CAD build for the part. Positions are in the model's coordinates, mm. A direction names the side the tool comes from. Round coordinates to 2 decimals unless told otherwise and drop trailing zeros. Order: outer loops, then holes, each group sorted by start corner. A loop starts at its lowest first (then second) coordinate and runs counter-clockwise, first axis right, second up. Notation, with made-up numbers: (71, -7) - (92, -7) arc R18 ccw to (92, 15) - close; hole circle Ø6 at (56, 12.25). An arc over 180 degrees is marked (long way). Use one line per item in the form item = value. Start each with the question number.
Autodesk Inventor part; units mm, degrees
ref_plane "YZ Plane" through (0, 0, 0) normal (1, 0, 0) x (0, 1, 0)
ref_plane "XZ Plane" through (0, 0, 0) normal (0, 1, 0) x (-1, 0, 0)
ref_plane "XY Plane" through (0, 0, 0) normal (0, 0, 1) x (1, 0, 0)
sketch "Sketch1" plane through (0, 0, 0) normal (0, 0, 1) x (1, 0, 0)
  line L0 (-3.0704, 18.7151) -> (-3.0704, 6.0151)
  line L1 (-3.0704, 6.0151) -> (-6.8804, 6.0151)
  line L2 (-6.8804, 6.0151) -> (-6.8804, -10.4949)
  line L3 (-6.8804, -10.4949) -> (-3.0704, -10.4949)
  line L4 (-3.0704, -10.4949) -> (-3.0704, -16.8449)
  line L5 (-3.0704, -16.8449) -> (-1.8004, -16.8449)
  line L6 (-1.8004, 18.7151) -> (-3.0704, 18.7151)
  line L7 (-1.8004, 18.7151) -> (-1.8004, -16.8449)
  dimension "d0" = 16.51
  dimension "d1" = 12.7
  dimension "d3" = 1.27
  dimension "d8" = 5.08
  dimension "d9" = 6.35
revolve "Revolution1" add sketch "Sketch1" angle 360 about axis through (-1.8004, 18.7151, 0) along (0, -1, 0)
properties part number "roll1"
(1) Which spindle directions (+Z, -Z, +X, -X, +Y, -Y) get a long thin tool onto all of the face, cutting with end or side? Do faces 1 (the cylindrical face through (-1.64, 12.28, -1.26)), 2 (the cylindrical face through (1.944, -2.355, -3.433)), 3 (the cylindrical face through (-1.64, -13.71, -1.26)). Say none if no direction does.
(2) Flat gauge pins, fed straight in: P1, Ø3, axis at x = -4.5, z = -2.5, coming from the +Y side; P2, Ø3, axis at y = 5.5, z = 3, coming from the +X side; P3, Ø2, axis at x = -5, z = 1.5, coming from the -Y side. Where does each tip first touch, or does it go through?
(3) Slice it at D-D (y = -6.5). Give the cut face in (x, z), and give its area (3 significant figures).
(4) Slice it at C-C (y = -13). Give the cut face in (x, z).
(5) Slice it at A-A (z = 0). Give the cut face in (x, y), and give its area (3 significant figures).
(6) Wall check: line 1 (Y direction, x = -3.5, z = 2.75); line 2 (Z direction, x = -1.75, y = 10.5); line 3 (X direction, y = 2, z = 0.25). Give the ranges that are in metal, low to high. Write a range as [from, to].
(7) Slice it at B-B (x = -1). Give the cut face in (y, z).
Results list:
q1.face_1 = +Y
q1.face_2 = +Y, -Y
q1.face_3 = -Y
q2.P1 = 6.02
q2.P2 = 3.05
q2.P3 = -10.49
q3.outline = circle Ø10.16 at (-1.8, 0)
q3.area = 81.1 mm²
q4.outline = circle Ø2.54 at (-1.8, 0)
q5.outline = (-6.88, -10.49) - (-3.07, -10.49) - (-3.07, -16.84) - (-0.53, -16.84) - (-0.53, -10.49) - (3.28, -10.49) - (3.28, 6.02) - (-0.53, 6.02) - (-0.53, 18.72) - (-3.07, 18.72) - (-3.07, 6.02) - (-6.88, 6.02) - close
q5.area = 216 mm²
q6.line_1 = [-10.49, 6.02]
q6.line_2 = [-1.27, 1.27]
q6.line_3 = [-6.87, 3.27]
q7.outline = (-16.84, -0.99) - (-10.49, -0.99) - (-10.49, -5.02) - (6.02, -5.02) - (6.02, -0.99) - (18.72, -0.99) - (18.72, 0.99) - (6.02, 0.99) - (6.02, 5.02) - (-10.49, 5.02) - (-10.49, 0.99) - (-16.84, 0.99) - close
